Part model, mm, in its own coordinate system. A direction names the side the tool comes from. Coordinates: 2 decimals unless noted, no trailing zeros. Loops run counter-clockwise (first coordinate to the right, second up) from the corner with the lowest first, then second, coordinate; pieces in that order, holes last. Notation, with made-up numbers: (81, -11) -> (106, -11) arc R33 cw to (106, 17) -> close; hole circle Ø7 at (-6.5, 78.25). An arc over 180 degrees is marked (long way). One line per question, with ' | ' between items. Start each with the question number.
1) 3-axis set-ups, long thin cutter, end or side, ignore diameter. For faces 1 (the face through (101, 155, 0)), 2 (the face through (99, 1, 2)), 3 (the face through (99, 203, 2)), 4 (the face through (101, 0, 15)): which of +Z, -Z, +X, -X, +Y, -Y reach the whole face in a straight line?
2) Two-plate mould, pull along Y, no slides. Class faces 5 (the face through (220, 51, 15)), 6 (the face through (209, 204, -1)), 7 (the face through (101, 100, 15)): released by +Y, released by -Y, zero draft, split by the parting line, or undercut.
3) Cut at B-B (y = 74.5). List the corners of the cut face in (x, z), plus the area to 3 significant figures.
4) Cut at C-C (z = 21.5). List the corners of the cut face in (x, y), plus the area to 3 significant figures.
5) Cut at A-A (x = 186). List the corners of the cut face in (y, z), plus the area to 3 significant figures.
6) Probe L1, parallel to Y at x = 157, z = 22.5; L2, parallel to Z at x = 46, y = 174; L3, parallel to Y at x = 146, z = 26.5. List the from-to ranges inside material, lowest first. Write a range as from..to.
7) Drop flat-ended pins along their axis: pin 1 (10 mm diameter, centred on x = 58, z = 13, fed in from -Y); pin 2 (1 mm diameter, centred on x = 135.5, y = 84, fed in from -Z); pin 3 (1.5 mm diameter, centred on x = 41.5, y = 84.5, fed in from +Z). Give the stop position or say it passes through.
from build123d import *

# Parameters (mm, degrees)
F0_W     = 100
F0_H     = 30
F1_DEPTH = 100
F2_W     = 104
F2_H     = 34
F2_W_2   = 100
F2_H_2   = 30
F3_DEPTH = 20
F4_R     = 5
F6_R     = 2.5


with BuildPart() as f1:
    # F0 (on Right) → F1 (new body)
    with BuildSketch(Plane.YZ):
        with Locations((50, 15)):
            Rectangle(F0_W, F0_H)
    extrude(amount=F1_DEPTH)

    # F2 (on face) → F3 (join)
    with BuildSketch(Plane(origin=(0, 0, 0), x_dir=(0, -1, 0), z_dir=(-1, 0, 0))):
        with Locations((-50, 15)):
            Rectangle(F2_W, F2_H)
        with Locations((-50, 15)):
            Rectangle(F2_W_2, F2_H_2, mode=Mode.SUBTRACT)
        with Locations((-50, 15)):
            Rectangle(F2_W_2, F2_H_2)
    extrude(amount=F3_DEPTH)

    # F4
    f4_edges = [f1.edges().sort_by_distance(p)[0] for p in [
        (50, 0, 30),
        (50, 0, 0),
        (50, 100, 30),
        (50, 100, 0),
        (-10, 102, 32),
        (-10, 102, -2),
        (-10, -2, 32),
        (-10, -2, -2),
    ]]
    fillet(f4_edges, radius=F4_R)

    # F5: F1 across face


with BuildPart() as f1_1:
    add(f1.part)
    add(f1.part.mirror(Plane(origin=(100, 50, 15), x_dir=(0, 1, 0), z_dir=(1, 0, 0))))

    # F6
    f6_edges = [f1_1.edges().sort_by_distance(p)[0] for p in [
        (-20, 50, 32),
        (-20, -0.535534, 30.535534),
        (-20, 100.535534, 30.535534),
        (-20, -2, 15),
        (-20, 102, 15),
        (-20, -0.535534, -0.535534),
        (-20, 100.535534, -0.535534),
        (-20, 50, -2),
        (220, 50, 32),
        (220, -0.535534, 30.535534),
        (220, 100.535534, 30.535534),
        (220, -2, 15),
        (220, 102, 15),
        (220, -0.535534, -0.535534),
        (220, 100.535534, -0.535534),
        (220, 50, -2),
    ]]
    fillet(f6_edges, radius=F6_R)

    # F7: F1 across face


with BuildPart() as f1_2:
    add(f1_1.part)
    add(f1_1.part.mirror(Plane(origin=(-8.75, 102, 15), x_dir=(-1, 0, 0), z_dir=(0, 1, 0))))


solid = f1_2.part
Reported:
1) face 1: -Z, +Y, -Y | face 2: -Z, -Y | face 3: -Z, +Y | face 4: +Z, -Z, -Y
2) face 5: zero draft | face 6: released by +Y | face 7: undercut
3) outline: (-20, 0.5) arc R2.5 ccw to (-17.5, -2) -> (0, -2) -> (0, 0) -> (200, 0) -> (200, -2) -> (217.5, -2) arc R2.5 ccw to (220, 0.5) -> (220, 29.5) arc R2.5 ccw to (217.5, 32) -> (200, 32) -> (200, 30) -> (0, 30) -> (0, 32) -> (-17.5, 32) arc R2.5 ccw to (-20, 29.5) -> close | area: 7,350 mm²
4) outline: (-20, 0.5) arc R2.5 ccw to (-17.5, -2) -> (0, -2) -> (0, 0) -> (200, 0) -> (200, -2) -> (217.5, -2) arc R2.5 ccw to (220, 0.5) -> (220, 99.5) arc R2.5 ccw to (217.5, 102) arc R2.5 ccw to (220, 104.5) -> (220, 203.5) arc R2.5 ccw to (217.5, 206) -> (200, 206) -> (200, 204) -> (0, 204) -> (0, 206) -> (-17.5, 206) arc R2.5 ccw to (-20, 203.5) -> (-20, 104.5) arc R2.5 ccw to (-17.5, 102) arc R2.5 ccw to (-20, 99.5) -> close; hole (0, 100) -> (200, 100) -> (200, 104) -> (0, 104) -> close | area: 48,300 mm²
5) outline: (0, 5) arc R5 ccw to (5, 0) -> (95, 0) arc R5 ccw to (100, 5) -> (100, 25) arc R5 ccw to (95, 30) -> (5, 30) arc R5 ccw to (0, 25) -> close; (104, 5) arc R5 ccw to (109, 0) -> (199, 0) arc R5 ccw to (204, 5) -> (204, 25) arc R5 ccw to (199, 30) -> (109, 30) arc R5 ccw to (104, 25) -> close | area: 5,960 mm²
6) L1: y = 0..100, 104..204 | L2: z = 0..30 | L3: y = 0.23..99.77, 104.23..203.77
7) pin 1: stops at y = 0 | pin 2: stops at z = 0 | pin 3: stops at z = 30
